Can you work these out from the model? Positions are in its coordinate system, mm. A direction names the side the tool comes from. Give positions to 0.01 mm unless a question says otherwise; leave off trailing zeros. Write each loop counter-clockwise with the first axis right and the second up, starting at its lowest first coordinate (ties: lowest second). Pieces come first, ordered by that corner, then holes.
1. Suppose I cut it at D-D (x = 33.5). Please give me the cut outline in (y, z), and give its area (3 significant figures).
2. Suppose I cut it at B-B (x = 11). Please give me the cut outline in (y, z).
3. Thinking about a two-plate mould opening in Y: for faces 4 (the flat face through (42.5, 3, -3)), 5 (the cylindrical face through (46.096, -0.044, -2.726)), 6 (the cylindrical face through (39.965, -12.203, 2.71)), which applies, pulls with the +Y half, pulls with the -Y half, needs draft (parallel to the pull), parting line crosses it, or undercut?
4. If I drill on probe 1 along X at (y, z) = (0, 0); probe 2 along Y at (x, z) = (25.5, -24); probe 3 along Y at (x, z) = (26, -5), over which ranges is the centre line in solid material (lowest first)?
5. On a 3-axis mill with a long thin cutter (end or side, diameter ignored), from which of +Z, -Z, +X, -X, +Y, -Y can I reach the whole of each face in a straight line? I mean faces 1 (the flat face through (37.5, 11.5, 5.9)), 2 (the flat face through (2.5, 0, 0)), 3 (the cylindrical face through (9.965, -12.203, 2.71)). Say none if no direction works.
6. I'm going to push flat-ended pins straight in: pin 1 (15 mm diameter, centred on y = -11, z = 5, fed in from +X); pin 2 (1.8 mm diameter, centred on x = 45.1, y = 0, fed in from +Z); pin 3 (10 mm diameter, centred on y = -0.5, z = 28.5, fed in from +X); pin 4 (3 mm diameter, centred on x = 45.1, y = 0, fed in from +Z). Where does each tip first touch, or does it pass through?
7. Suppose I cut it at A-A (z = 0). Give the number of separate pieces and of enclosed holes in the cut face, and give its area (3 significant figures).
```python
from build123d import *

# Parameters (mm, degrees)
IZIM1_R                          = 75
IZIM1_R_2                        = 25
Y_KSEKLIK_EKSTR_ZYON2_DEPTH      = 50
RADYUS2_R                        = 25
Y_KSEKLIK_EKSTR_ZYON3_DEPTH      = 60
Y_KSEKLIK_EKSTR_ZYON3_DEPTH_BACK = 10
IZIM2_R                          = 25
IZIM3_R                          = 7.5
Y_KSEKLIK_EKSTR_ZYON5_DEPTH      = 10
KES_EKSTR_ZYON1_DEPTH            = 10
KES_EKSTR_ZYON1_DEPTH_BACK       = 10
IZIM4_R                          = 4
Y_KSEKLIK_EKSTR_ZYON6_START      = 10
IZIM5_R                          = 7.5
Y_KSEKLIK_EKSTR_ZYON6_DEPTH      = 10
KES_EKSTR_ZYON2_DEPTH            = 10
KES_EKSTR_ZYON2_DEPTH_BACK       = 10
IZIM6_R                          = 4
KES_EKSTR_ZYON3_DEPTH            = 10
KES_EKSTR_ZYON3_DEPTH_BACK       = 10
IZIM7_R                          = 2
KES_EKSTR_ZYON4_DEPTH            = 10
KES_EKSTR_ZYON4_DEPTH_BACK       = 10
IZIM8_R                          = 2
L_EK2_SCALE                      = 0.5


with BuildPart() as part:
    # Çizim1 → Yükseklik-Ekstrüzyon2 (new body)
    with BuildSketch(Plane(origin=(0, 0, 0), x_dir=(0, 0, -1), z_dir=(1, 0, 0))):
        Circle(IZIM1_R)
        Circle(IZIM1_R_2, mode=Mode.SUBTRACT)
    extrude(amount=Y_KSEKLIK_EKSTR_ZYON2_DEPTH)

    # Radyus2
    radyus2_edges = [part.edges().sort_by_distance(p)[0] for p in [
        (0, 0, 75),
        (50, 0, 75),
    ]]
    fillet(radyus2_edges, radius=RADYUS2_R - 0.0001)  # a hair under: the kernel refuses the full size

    # Çizim2 → Yükseklik-Ekstrüzyon3 (add, two sides: drawn at the far end of the back side and taken through both)
    with BuildSketch(Plane(origin=(0, 0, 0), x_dir=(0, 0, -1), z_dir=(1, 0, 0)).offset(-Y_KSEKLIK_EKSTR_ZYON3_DEPTH_BACK)):
        Circle(IZIM2_R)
    extrude(amount=Y_KSEKLIK_EKSTR_ZYON3_DEPTH + Y_KSEKLIK_EKSTR_ZYON3_DEPTH_BACK)

    # Çizim3 → Yükseklik-Ekstrüzyon5 (add)
    with BuildSketch(Plane(origin=(60, 0, 0), x_dir=(0, 0, -1), z_dir=(1, 0, 0))):
        Circle(IZIM3_R)
    extrude(amount=Y_KSEKLIK_EKSTR_ZYON5_DEPTH)

    # Çizim4 → Kes-Ekstrüzyon1 (cut, two sides: drawn at the far end of the back side and taken through both)
    with BuildSketch(Plane(origin=(0, 0, 0), x_dir=(1, 0, 0), z_dir=(0, 1, 0)).offset(-KES_EKSTR_ZYON1_DEPTH_BACK)):
        with Locations(Location((65, 0, 0), (0, 0, 90))):
            Circle(IZIM4_R)
    extrude(amount=KES_EKSTR_ZYON1_DEPTH + KES_EKSTR_ZYON1_DEPTH_BACK, mode=Mode.SUBTRACT)

    # Çizim5 → Yükseklik-Ekstrüzyon6 (add)
    with BuildSketch(Plane.ZY.offset(10).offset(Y_KSEKLIK_EKSTR_ZYON6_START)):
        with Locations(Location((0, 0, 0), (0, 0, 180))):
            Circle(IZIM5_R)
    extrude(amount=-Y_KSEKLIK_EKSTR_ZYON6_DEPTH)

    # Çizim6 → Kes-Ekstrüzyon2 (cut, two sides: drawn at the far end of the back side and taken through both)
    with BuildSketch(Plane(origin=(0, 0, 0), x_dir=(1, 0, 0), z_dir=(0, 1, 0)).offset(-KES_EKSTR_ZYON2_DEPTH_BACK)):
        with Locations(Location((-15, 0, 0), (0, 0, 90))):
            Circle(IZIM6_R)
    extrude(amount=KES_EKSTR_ZYON2_DEPTH + KES_EKSTR_ZYON2_DEPTH_BACK, mode=Mode.SUBTRACT)

    # Çizim7 → Kes-Ekstrüzyon3 (cut, two sides: drawn at the far end of the back side and taken through both)
    with BuildSketch(Plane.XY.offset(-KES_EKSTR_ZYON3_DEPTH_BACK)):
        with Locations(Location((65.194673775, 0, 0), (0, 0, 180))):
            Circle(IZIM7_R)
    extrude(amount=KES_EKSTR_ZYON3_DEPTH + KES_EKSTR_ZYON3_DEPTH_BACK, mode=Mode.SUBTRACT)

    # Çizim8 → Kes-Ekstrüzyon4 (cut, two sides: drawn at the far end of the back side and taken through both)
    with BuildSketch(Plane.XY.offset(-KES_EKSTR_ZYON4_DEPTH_BACK)):
        with Locations(Location((-15.164276084, 0, 0), (0, 0, 180))):
            Circle(IZIM8_R)
    extrude(amount=KES_EKSTR_ZYON4_DEPTH + KES_EKSTR_ZYON4_DEPTH_BACK, mode=Mode.SUBTRACT)


with BuildPart() as part_1:
    # Ölçek2: scaled about (24.999995203, 7e-09, 5.8e-08)
    add(part.part.scale(L_EK2_SCALE).moved(Location((12.499997602, 3e-09, 2.9e-08))))


solid = part_1.part
```
Checks:
1. outline: circle Ø68.33 at (0, 0)
1. area: 3,670 mm2
2. outline: circle Ø25 at (0, 0)
3. face 4: needs draft
3. face 5: undercut
3. face 6: parting line crosses it
4. probe 1: x = 2.5 to 3, 7 to 43, 47 to 47.5
4. probe 2: y = -28.8 to 28.8
4. probe 3: y = -37.12 to 37.12
5. face 1: +X
5. face 2: +Z, -Z, -X, +Y, -Y
5. face 3: -X
6. pin 1: stops at x = 42.5
6. pin 2: passes through
6. pin 3: stops at x = 37.5
6. pin 4: stops at z = 3.75
7. separate pieces: 3
7. enclosed holes: 0
7. area: 2,010 mm2
